Geometry check sheet. Reference: drawing and pictorial views, mm from the part's lowest x, y, z. Coordinates: 2 decimals unless noted, no trailing zeros. Loops run counter-clockwise (first coordinate to the right, second up) from the corner with the lowest first, then second, coordinate; pieces in that order, holes last. Notation, with made-up numbers: (27, 73) - (47, 73) arc R21 ccw to (47, 90) - close; hole circle Ø2 at (61, -6). An arc over 180 degrees is marked (long way). One line per item, written item: value.
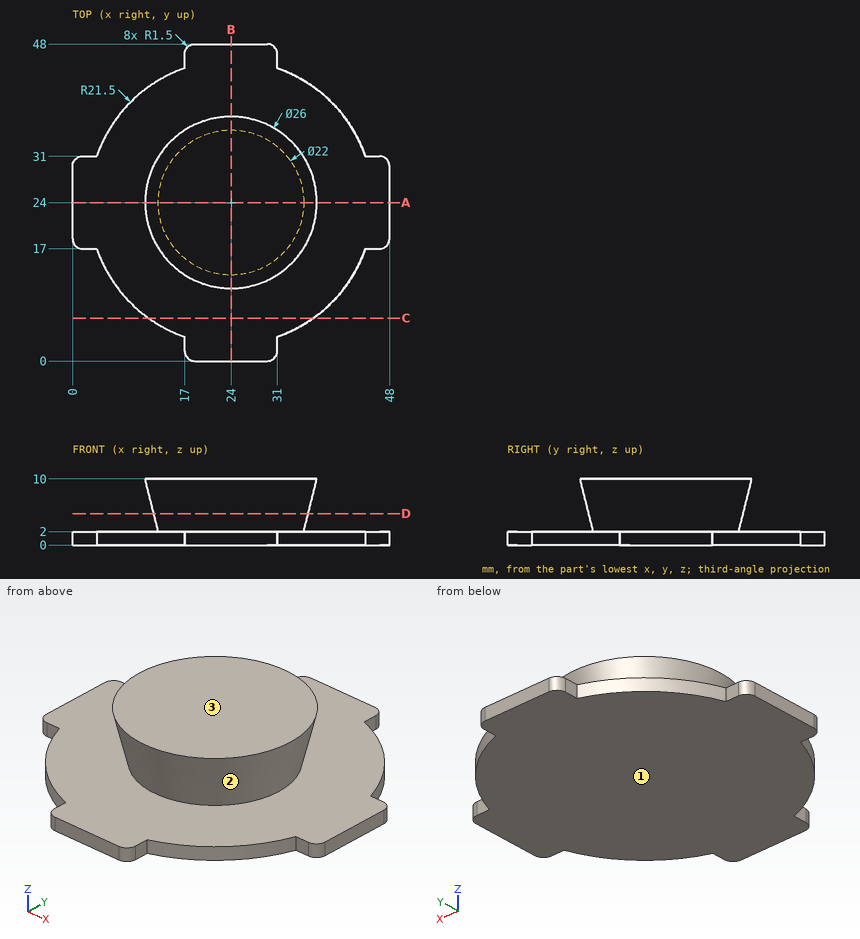
(1) Cross-section at A-A on y = 24. Record the cut outline in (x, z).
Reply:
outline: (0, 0) - (48, 0) - (48, 2) - (35, 2) - (37, 10) - (11, 10) - (13, 2) - (0, 2) - close
(2) Cross-section at C-C on y = 6.5. Record the cut outline in (x, z), and give its area (3 significant figures).
Reply:
outline: (11.51, 0) - (36.49, 0) - (36.49, 2) - (11.51, 2) - close
area: 50.0 mm2
(3) Release check for a two-part mould opening along Z. For the marked faces 1, 2 and 3 record: pulls with the +Z half, pulls with the -Z half, needs draft (parallel to the pull), parting line crosses it, or undercut.
Reply:
face 1: pulls with the -Z half
face 2: undercut
face 3: pulls with the +Z half
(4) Cross-section at D-D on z = 4.75. Record the cut outline in (x, y) (1 decimal), and give its area (3 significant figures).
Reply:
outline: circle Ø23.4 at (24, 24)
area: 429 mm2
(5) Go/stop test with flat-tipped pins: pin 1 Ø5 at (x, z) = (13.5, 8) entering from +Y; pin 2 Ø1 at (y, z) = (45.5, 0.5) entering from +X; pin 3 Ø1.6 at (x, z) = (2.5, 1) entering from +Y; pin 4 Ø4 at (x, z) = (39.5, 9) entering from -Y. Record where each tip stops, or that it passes through.
Reply:
pin 1: y = 33.76
pin 2: x = 31
pin 3: y = 31
pin 4: through
(6) Material ranges on probe 1 along Z at (x, y) = (38, 9.5); probe 2 along X at (y, z) = (23.5, 8); probe 3 along X at (y, z) = (29, 9), recorded low to high. Write a range as from..to.
Reply:
probe 1: 0..2
probe 2: 11.51..36.49
probe 3: 12.27..35.73
